Work out the finished part from the listing and answer in its coordinate system (mm). A direction names the side the tool comes from. Coordinates: 2 decimals unless noted, no trailing zeros. Write each loop counter-clockwise with the first axis right and the second up, starting at its lowest first coordinate (ties: lowest second). Pieces come first, ordered by that corner, then holes. Notation, with made-up numbers: (86.5, 35.25) - (99.5, 35.25) arc R21 cw to (99.5, 57.25) - close; hole circle Ø4 at (8.25, 1.5). An arc over 180 degrees is marked (long way). Answer as a JSON object with one key per item and string values. Group by question number.
from build123d import *

# Parameters (mm, degrees)
F0_W     = 80
F0_H     = 8
F0_R     = 1.5
F1_DEPTH = 7
F2_R     = 3.99999
F3_W     = 25
F3_H     = 20
F4_DEPTH = 2
F6_DEPTH = 1.3
F8_DEPTH = 2
F9_D     = 3.2
F9_DEPTH = 6
F9_TIP   = 0.9613769904


# Not quite as in the source:
# - a fillet or chamfer is up to 0.001 mm smaller than in the source, because OpenCascade refuses the exact size


with BuildPart() as f1:
    # F0 (on Top) → F1 (new body)
    with BuildSketch(Plane.XY):
        with Locations((-23.5758614609, 11.990132276)):
            Rectangle(F0_W, F0_H)
        with Locations((-59.5758614609, 11.990132276)):
            Circle(F0_R, mode=Mode.SUBTRACT)
    extrude(amount=F1_DEPTH)

    # F2 (radius 4 in the source; OpenCascade refuses exactly that, so slightly less here)
    f2_edges = [f1.edges().sort_by_distance(p)[0] for p in [
        (-63.575861, 15.990132, 3.5),
        (-63.575861, 7.990132, 3.5),
    ]]
    fillet(f2_edges, radius=F2_R)

    # F3 (on face) → F4 (join)
    with BuildSketch(Plane.YZ.offset(16.4241385391)):
        with Locations((11.990132276, 10)):
            Rectangle(F3_W, F3_H)
    extrude(amount=F4_DEPTH)

    # F5 (on face) → F6 (join)
    with BuildSketch(Plane.YZ.offset(18.4241385391)):
        Polygon((1.490132276, 9), (-0.509867724, 9), (-0.509867724, 0), (24.490132276, 0), (24.490132276, 9), (22.490132276, 9), (22.490132276, 2), (1.490132276, 2), align=None)
    extrude(amount=F6_DEPTH)

    # F7 (on face) → F8 (join)
    with BuildSketch(Plane.YZ.offset(19.7241385391)):
        Polygon((11.290132276, 9), (-0.509867724, 9), (-0.509867724, 0), (24.490132276, 0), (24.490132276, 9), (12.690132276, 9), (12.690132276, 2), (11.290132276, 2), align=None)
    extrude(amount=F8_DEPTH)

    # F9
    with Locations(Plane(origin=(16.4241385391, 0, 0), x_dir=(0, 1, 0), z_dir=(-1, 0, 0))):
        with Locations((2.490132276, -17), (21.490132276, -17)):
            Hole(F9_D / 2, depth=F9_DEPTH)
            with Locations((0, 0, -(F9_DEPTH + F9_TIP / 2))):  # 118° drill point
                Cone(0, F9_D / 2, F9_TIP, mode=Mode.SUBTRACT)


solid = f1.part
Q1. A tool of negligible diameter and unlimited length cuts with its end or side. For faces 4 (the face through (21, 11.29, 5)), 5 (the face through (21, 5, 9)), 6 (the face through (-24, 12, 7)), 7 (the face through (19.724, 18, 6)), from which of +Z, -Z, +X, -X, +Y, -Y can it reach the whole face along a straight path? Write none if from no direction.
Q2. Section D-D on y = 3.25 is taken. Determine the outline of the cut face in (x, z).
Q3. For a pull along Y with two mould halves and no side action, classify faces 1 (the face through (16.424, 12, 10)), 2 (the face through (-62.435, 14.787, 3.549)), 3 (the face through (17.438, 2.698, 15.414)) as +Y half, -Y half, draft (parallel to the pull), parting line (faces both ways), or undercut.
Q4. Consider L1, parallel to Y at x = 17.6, z = 17; L2, parallel to X at y = 3.5, z = 14.5; L3, parallel to X at y = 20.75, z = 1.75. Determine where each line is inside the solid, lowest interval first. Write a range as from..to.
Q5. Flat-ended cylindrical pins translate along their axes: pin 1 Ø1 at (x, y) = (19.5, 5) entering from +Z; pin 2 Ø7.5 at (x, z) = (-36, 2) entering from -Y; pin 3 Ø12 at (y, z) = (12.5, 15) entering from -X. Find the tip coordinate at first contact, or state that the pin passes through.
Q6. Section B-B on y = 19 is taken. Determine the outline of the cut face in (x, z), plus the area to 3 significant figures.
Q7. Section A-A on z = 17 is taken. Determine the outline of the cut face in (x, y).
Numbers:
{
 "1": {"face 4": "+Z, +X", "face 5": "+Z, +X, +Y, -Y", "face 6": "+Z, -X, +Y, -Y", "face 7": "+Z"},
 "2": {"outline": "(16.42, 0) - (21.72, 0) - (21.72, 9) - (19.72, 9) - (19.72, 2) - (18.42, 2) - (18.42, 15.59) - (16.42, 15.59) - close; (16.42, 18.41) - (18.42, 18.41) - (18.42, 20) - (16.42, 20) - close"},
 "3": {"face 1": "draft", "face 2": "+Y half", "face 3": "undercut"},
 "4": {"L1": "y = -0.51..0.89, 4.09..19.89, 23.09..24.49", "L2": "x = 16.42..18.42", "L3": "x = 16.42..21.72"},
 "5": {"pin 1": "stops at z = 9", "pin 2": "stops at y = 7.99", "pin 3": "stops at x = 16.42"},
 "6": {"outline": "(16.42, 0) - (21.72, 0) - (21.72, 9) - (19.72, 9) - (19.72, 2) - (18.42, 2) - (18.42, 20) - (16.42, 20) - close", "area": "60.6 mm²"},
 "7": {"outline": "(16.42, -0.51) - (18.42, -0.51) - (18.42, 0.89) - (16.42, 0.89) - close; (16.42, 4.09) - (18.42, 4.09) - (18.42, 19.89) - (16.42, 19.89) - close; (16.42, 23.09) - (18.42, 23.09) - (18.42, 24.49) - (16.42, 24.49) - close"}
}
